from build123d import *

# Parameters (mm, degrees)
BOSS_EXTRUDE1_DEPTH       = 5
BOSS_EXTRUDE2_DEPTH       = 5
FILLET2_R                 = 5
SKETCH2_R                 = 3
CUT_EXTRUDE1_DEPTH        = 225.405408442
SKETCH4_R                 = 3
CUT_EXTRUDE2_DEPTH        = 225.405408442
SKETCH5_R                 = 1.25
CUT_EXTRUDE3_DEPTH        = 225.405408442
SKETCH8_R                 = 1.25
CUT_EXTRUDE4_DEPTH        = 225.405408442
BOSS_EXTRUDE3_DEPTH       = 5
SKETCH15_R                = 2
CUT_EXTRUDE8_DEPTH        = 225.405408442
SKETCH17_R                = 1.5
CUT_EXTRUDE9_DEPTH        = 3
SKETCH19_R                = 4
CUT_EXTRUDE11_DEPTH       = 225.405408444
M2X0_4_TAPPED_HOLE2_D     = 1.6
M4X0_7_TAPPED_HOLE1_D     = 3.3
M4X0_7_TAPPED_HOLE1_DEPTH = 11.5
M4X0_7_TAPPED_HOLE1_TIP   = 0.991420021


with BuildPart() as part:
    # Sketch1 → Boss-Extrude1 (new body)
    with BuildSketch(Plane.XY):
        with BuildLine():
            Line((-12.5, 0), (-12.5, -78.5))
            Line((-12.5, -78.5), (-17.5, -78.5))
            Line((-17.5, -78.5), (-17.5, -106.384985834))
            Line((-17.5, -106.384985834), (-96.852760713, -168.992385615))
            ThreePointArc((-96.852760713, -168.992385615), (-112.63340609, -187.366759998), (-89.969843477, -178.822210146))
            Line((-89.969843477, -178.822210146), (-11.841670305, -130.517603057))
            ThreePointArc((-11.841670305, -130.517603057), (-6.105731879, -132.742937904), (0, -133.5))
            Line((0, -133.5), (0, -108.5))
            Line((0, -108.5), (0, 0))
            Line((0, 0), (0, 12.5))
            ThreePointArc((0, 12.5), (-8.838834765, 8.838834765), (-12.5, 0))
        make_face()
    extrude(amount=BOSS_EXTRUDE1_DEPTH)

    # Sketch3 → Boss-Extrude2 (add)
    with BuildSketch(Plane.XY):
        with BuildLine():
            Line((-22.5, 59.99791663), (0, 0))
            Line((0, 0), (-12.5, 0))
            Line((-12.5, 0), (-12.5, 23.076121781))
            Line((-12.5, 23.076121781), (-32.5, 59.99791663))
            Line((-32.5, 59.99791663), (-6.274365114, 105.186702896))
            ThreePointArc((-6.274365114, 105.186702896), (-12.070421941, 119.246749368), (0, 128.49791663))
            Line((0, 128.49791663), (0, 115.99791663))
            Line((0, 115.99791663), (0, 90.99791663))
            ThreePointArc((0, 90.99791663), (-4.74657039, 91.452650905), (-9.320466521, 92.800311068))
            Line((-9.320466521, 92.800311068), (-22.5, 59.99791663))
        make_face()
    extrude(amount=BOSS_EXTRUDE2_DEPTH)

    # Fillet2
    fillet2_edges = [part.edges().sort_by_distance(p)[0] for p in [
        (-12.5, -78.5, 2.5),
    ]]
    fillet(fillet2_edges, radius=FILLET2_R - 0.0001)  # a hair under: the kernel refuses the full size

    # Mirror1: part across plane


with BuildPart() as part_1:
    add(part.part)
    add(part.part.mirror(Plane(origin=(0, -133.5, 5), x_dir=(0, 0, 1), z_dir=(-1, 0, 0))))

    # Sketch2 → Cut-Extrude1 (cut, through all)
    with BuildSketch(Plane.XY.offset(5)):
        with Locations((0, -108.5)):
            Circle(SKETCH2_R)
    extrude(amount=-CUT_EXTRUDE1_DEPTH, mode=Mode.SUBTRACT)

    # Sketch4 → Cut-Extrude2 (cut, through all)
    with BuildSketch(Plane.XY.offset(5)):
        with Locations((-102.394005536, -180.197054544)):
            Circle(SKETCH4_R)
        with Locations((102.394005536, -180.197054544)):
            Circle(SKETCH4_R)
        with Locations((0, 115.99791663)):
            Circle(SKETCH4_R)
    extrude(amount=-CUT_EXTRUDE2_DEPTH, mode=Mode.SUBTRACT)

    # Sketch5 → Cut-Extrude3 (cut, through all)
    with BuildSketch(Plane.XY.offset(5)):
        Circle(SKETCH5_R)
    extrude(amount=-CUT_EXTRUDE3_DEPTH, mode=Mode.SUBTRACT)

    # Sketch7 → Cut-Revolve2 (revolve, cut)
    with BuildSketch(Plane(origin=(0, 0, 0), x_dir=(0, 0, -1), z_dir=(1, 0, 0)), mode=Mode.PRIVATE) as cut_revolve2_sk:
        with BuildLine():
            Line((-5, 0), (-2, 0))
            ThreePointArc((-2, 0), (-2.878679656, -2.121320344), (-5, -3))
            Line((-5, -3), (-5, 0))
        make_face()
    cut_revolve2 = revolve(cut_revolve2_sk.sketch.rotate(Axis((0, 0, 5), (0, 0, -1)), 270), axis=Axis((0, 0, 5), (0, 0, -1)), mode=Mode.SUBTRACT)

    # Sketch8 → Cut-Extrude4 (cut, through all)
    with BuildSketch(Plane(origin=(0, 0, 0), x_dir=(-1, 0, 0), z_dir=(0, 0, -1))):
        with Locations((-27.5, 59.99791663)):
            Circle(SKETCH8_R)
        with Locations((27.5, 59.99791663)):
            Circle(SKETCH8_R)
    extrude(amount=-CUT_EXTRUDE4_DEPTH, mode=Mode.SUBTRACT)

    # Sketch14 → Boss-Extrude3 (add)
    with BuildSketch(Plane.XY.offset(5)):
        with BuildLine():
            Line((-3.5, 127.99791663), (3.5, 127.99791663))
            Line((3.5, 127.99791663), (3.5, 132.99791663))
            ThreePointArc((3.5, 132.99791663), (0, 133.354471588), (-3.5, 132.99791663))
            Line((-3.5, 132.99791663), (-3.5, 127.99791663))
        make_face()
    extrude(amount=-BOSS_EXTRUDE3_DEPTH)

    # Sketch15 → Cut-Extrude8 (cut, through all)
    with BuildSketch(Plane.XY.offset(5)):
        with Locations((0, 104.99791663)):
            Circle(SKETCH15_R)
        with Locations((0, 129.99791663)):
            Circle(SKETCH15_R)
    extrude(amount=-CUT_EXTRUDE8_DEPTH, mode=Mode.SUBTRACT)

    # Sketch17 → Cut-Extrude9 (cut)
    with BuildSketch(Plane(origin=(0, 133.354471588, 0), x_dir=(1, 0, 0), z_dir=(0, 1, 0))):
        with Locations(Location((0, -2.5, 0), (0, 0, 270))):
            Circle(SKETCH17_R)
    extrude(amount=-CUT_EXTRUDE9_DEPTH, mode=Mode.SUBTRACT)

    # Sketch19 → Cut-Extrude11 (cut, through all)
    with BuildSketch(Plane.XY.offset(5)):
        with Locations((1.5, 95.99791663)):
            Circle(SKETCH19_R)
    extrude(amount=-CUT_EXTRUDE11_DEPTH, mode=Mode.SUBTRACT)

    # M2x0.4 Tapped Hole2 (through all)
    with Locations(Plane(origin=(0, 0, 0), x_dir=(1, 0, 0), z_dir=(0, 0, -1))):
        with Locations((8.5, -95.99791663), (-5.5, -95.99791663)):
            Hole(M2X0_4_TAPPED_HOLE2_D / 2)

    # Sketch-Pattern1: Cut-Revolve2 at 2 more places
    with Locations((27.5, 59.997917, 0), (-27.5, 59.997917, 0)):
        add(cut_revolve2, mode=Mode.SUBTRACT)

    # M4x0.7 Tapped Hole1
    with Locations(Plane.XZ.offset(192.697054544)):
        with Locations((102.394005536, 2.5), (-102.394005536, 2.5)):
            Hole(M4X0_7_TAPPED_HOLE1_D / 2, depth=M4X0_7_TAPPED_HOLE1_DEPTH)
            with Locations((0, 0, -(M4X0_7_TAPPED_HOLE1_DEPTH + M4X0_7_TAPPED_HOLE1_TIP / 2))):  # 118° drill point
                Cone(0, M4X0_7_TAPPED_HOLE1_D / 2, M4X0_7_TAPPED_HOLE1_TIP, mode=Mode.SUBTRACT)


solid = part_1.part
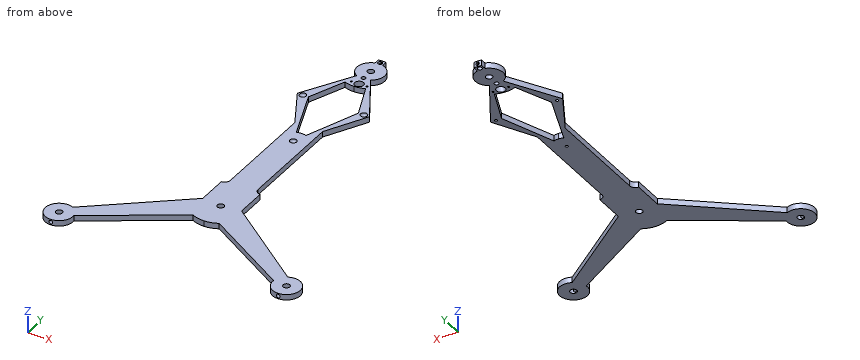
Can you work these out from the model? Positions are in its coordinate system, mm. Round coordinates to 2 decimals unless told otherwise and drop trailing zeros. Write each loop counter-clockwise with the first axis right and the second up, starting at its lowest first coordinate (ties: lowest second). Pieces come first, ordered by that corner, then holes. Notation, with made-up numbers: M 6,-31.75 L 55,-31.75 A13 cw 55,-22.75 Z; hole C 60.5,2 d5. An arc over 180 degrees is marked long. Use CSV: the item, a comma, the result in double quotes.
(1) Imagine slicing it at A-A (y = 75.5). Write out the boundary of the cut face in (x, z), plus the area to 3 significant figures.
Check values:
outline,"M -23.5,0 L -16.27,0 L -16.27,5 L -23.5,5 Z; M 16.27,0 L 23.5,0 L 23.5,5 L 16.27,5 Z"
area,"72.3 mm^2"
(2) Imagine slicing it at B-B (y = -31.5). Write out the boundary of the cut face in (x, z).
Check values:
outline,"M -12.5,0 L 12.5,0 L 12.5,5 L -12.5,5 Z"
(3) I'm going to push flat-ended pins straight in: pin 1 (1.5 mm diameter, centred on y = 131, z = 1.5, fed in from -X); pin 2 (1.5 mm diameter, centred on y = -34, z = 2.5, fed in from -X). Where does each tip first touch, or does it pass through?
Check values:
pin 1,"x = -3.5"
pin 2,"x = -12.5"
(4) I need wall thicknesses on line 1 along X through (y, z) = (-187, 2.5); line 2 along X through (y, z) = (46.5, 4.6); line 3 along X through (y, z) = (68.5, 3.65). Which ranges of each line are inside material? Lowest first, please.
Check values:
line 1,"-112.88 to -104.04, -100.74 to -91.91, 91.91 to 100.74, 104.04 to 112.88"
line 2,"-25.19 to -17.44, 17.44 to 25.19"
line 3,"-27.57 to -19.08, 19.08 to 27.57"
(5) Imagine slicing it at C-C (y = 27). Write out the boundary of the cut face in (x, z), plus the area to 3 significant figures.
Check values:
outline,"M -14.63,0 L -10.13,0 L -10.13,5 L -14.63,5 Z; M 10.13,0 L 14.63,0 L 14.63,5 L 10.13,5 Z"
area,"45.0 mm^2"
